```python
from build123d import *

# Parameters (mm, degrees)
SKETCH1_R           = 3.95
BOSS_EXTRUDE1_DEPTH = 6
CHAMFER1_SIZE       = 0.25


with BuildPart() as part:
    # Sketch1 → Boss-Extrude1 (new, symmetric)
    with BuildSketch(Plane(origin=(0, 0, 0), x_dir=(1, 0, 0), z_dir=(0, 1, 0))):
        with Locations(Location((0, 0, 0), (0, 0, 270))):
            Circle(SKETCH1_R)
    extrude(amount=BOSS_EXTRUDE1_DEPTH, both=True)

    # Sketch2 → Revolve2 (revolve)
    with BuildSketch(Plane.XY, mode=Mode.PRIVATE) as revolve2_sk:
        Polygon((0, -10.5), (0, -6), (-3.95, -6), (-3.9, -6.15), (-3.9, -10.5), align=None)
        Polygon((0, 10.5), (0, 6), (3.95, 6), (3.9, 6.125), (3.9, 10.5), align=None)
    revolve(revolve2_sk.sketch.rotate(Axis((0, -10.5, 0), (0, 1, 0)), 180), axis=Axis((0, -10.5, 0), (0, 1, 0)))

    # Chamfer1
    chamfer1_edges = [part.edges().sort_by_distance(p)[0] for p in [
        (-3.9, -10.5, 0),
        (3.9, 10.5, 0),
    ]]
    chamfer(chamfer1_edges, length=CHAMFER1_SIZE)


solid = part.part
```
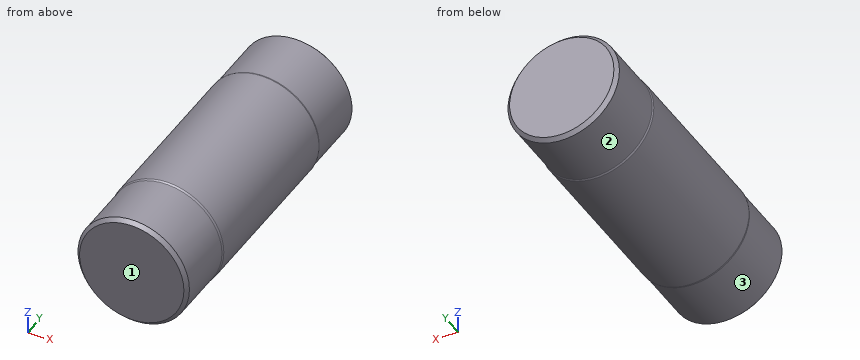
Geometry check sheet. Reference: the model listing, model coordinates, mm. Face numbers are marked on the shaded views. A direction names the side the tool comes from. Give positions to 0.01 mm unless a question says otherwise; leave off trailing zeros. Write each loop counter-clockwise with the first axis right and the second up, starting at its lowest first coordinate (ties: lowest second). Pieces come first, ordered by that corner, then holes.
1) Material ranges on L1, parallel to Y at x = 2.75, z = -2.5; L2, parallel to Z at x = 2.5, y = 8; L3, parallel to Z at x = -1, y = -5.25, recorded low to high.
2) Section check A-A, the plane y = 0.5. Record the boundary of the cut face in (x, z), and give its area (3 significant figures).
3) Access from +Z, -Z, +X, -X, +Y, -Y to the whole of each face (thin tool, end or side, straight path). Record for the marked faces 1, 2 and 3.
Computed:
1. L1: y = -10.43 to 10.43
1. L2: z = -2.99 to 2.99
1. L3: z = -3.82 to 3.82
2. outline: circle Ø7.9 at (0, 0)
2. area: 49.0 mm2
3. face 1: +Z, -Z, +X, -X, -Y
3. face 2: +Y
3. face 3: -Y
